Part model, mm, in its own coordinate system. Give positions to 0.01 mm unless a question says otherwise; leave off trailing zeros. Order: outer loops, then holes, each group sorted by start corner. A loop starts at its lowest first (then second) coordinate and runs counter-clockwise, first axis right, second up. Notation, with made-up numbers: M -30,51 L 19,51 A18 ccw 19,84 Z; hole C 50,51 d1. An arc over 180 degrees is marked long. Write each question's results on one line, items separated by ' | '. Start each with the question number.
from build123d import *

# Parameters (mm, degrees)
SKETCH1_R             = 41.5
MAIN_PLATE_DEPTH      = 5
SKETCH2_R             = 2.05
CUT_EXTRUDE_G27_DEPTH = 59.902461748
SKETCH3_R             = 2.5
MOMO_SPARKO_DEPTH     = 59.902461748
SKETCH4_R             = 17.5
CENTER_HOLE_DEPTH     = 59.902461748
FILLET1_R             = 2
FILLET2_R             = 2


with BuildPart() as part:
    # Sketch1 → Main Plate (new body)
    with BuildSketch(Plane(origin=(0, 0, 0), x_dir=(1, 0, 0), z_dir=(0, 1, 0))):
        with Locations(Location((0, 0, 0), (0, 0, 270))):
            Circle(SKETCH1_R)
    extrude(amount=MAIN_PLATE_DEPTH)

    # Sketch2 → Cut-Extrude G27 (cut, through all)
    with BuildSketch(Plane(origin=(0, 5, 0), x_dir=(1, 0, 0), z_dir=(0, 1, 0))):
        with Locations(Location((0, 27.5, 0), (0, 0, 270))):
            Circle(SKETCH2_R)
        with Locations(Location((23.815698604, 13.75, 0), (0, 0, 270))):
            Circle(SKETCH2_R)
        with Locations(Location((23.815698604, -13.75, 0), (0, 0, 270))):
            Circle(SKETCH2_R)
        with Locations(Location((0, -27.5, 0), (0, 0, 270))):
            Circle(SKETCH2_R)
        with Locations(Location((-23.815698604, -13.75, 0), (0, 0, 270))):
            Circle(SKETCH2_R)
        with Locations(Location((-23.815698604, 13.75, 0), (0, 0, 270))):
            Circle(SKETCH2_R)
    extrude(amount=-CUT_EXTRUDE_G27_DEPTH, mode=Mode.SUBTRACT)

    # Sketch3 → Momo - Sparko (cut, through all)
    with BuildSketch(Plane(origin=(0, 5, 0), x_dir=(1, 0, 0), z_dir=(0, 1, 0))):
        with Locations(Location((0, 35, 0), (0, 0, 270))):
            Circle(SKETCH3_R)
        with Locations(Location((30.310889132, 17.5, 0), (0, 0, 270))):
            Circle(SKETCH3_R)
        with Locations(Location((30.310889132, -17.5, 0), (0, 0, 270))):
            Circle(SKETCH3_R)
        with Locations(Location((0, -35, 0), (0, 0, 270))):
            Circle(SKETCH3_R)
        with Locations(Location((-30.310889132, -17.5, 0), (0, 0, 270))):
            Circle(SKETCH3_R)
        with Locations(Location((-30.310889132, 17.5, 0), (0, 0, 270))):
            Circle(SKETCH3_R)
    extrude(amount=-MOMO_SPARKO_DEPTH, mode=Mode.SUBTRACT)

    # Sketch4 → Center Hole (cut, through all)
    with BuildSketch(Plane(origin=(0, 5, 0), x_dir=(1, 0, 0), z_dir=(0, 1, 0))):
        with Locations(Location((0, 0, 0), (0, 0, 270))):
            Circle(SKETCH4_R)
    extrude(amount=-CENTER_HOLE_DEPTH, mode=Mode.SUBTRACT)

    # Fillet1
    fillet1_edges = [part.edges().sort_by_distance(p)[0] for p in [
        (0, 5, -41.5),
    ]]
    fillet(fillet1_edges, radius=FILLET1_R)

    # Fillet2
    fillet2_edges = [part.edges().sort_by_distance(p)[0] for p in [
        (0, 0, -41.5),
    ]]
    fillet(fillet2_edges, radius=FILLET2_R)


solid = part.part
(1) Drop flat-ended pins along their axis: P1, Ø1.5, axis at x = 29, y = 3.5, coming from the +Z side; P2, Ø8, axis at x = 0, z = -35, coming from the -Y side. Give the stop position or say it passes through.
(2) Probe L1, parallel to Z at x = -24.5, y = 4.3; L2, parallel to Z at x = -1.5, y = 1.9; L3, parallel to Z at x = -12, y = 4.75. List the from-to ranges inside material, lowest first.
(3) Saw through at B-B on x = 0. Give the cut face in (y, z).
(4) Saw through at A-A on z = 0. Give the cut face in (x, y), plus the area to 3 significant figures.
(5) Saw through at C-C on x = -31.5. Give the number of separate pieces and of enclosed holes in the cut face, plus the area to 3 significant figures.
(6) Pull direction Z, two halves, no side cores. Call faces 1 (the cylindrical face through (-32.75, 2.54, 16.96)), 2 (the cylindrical face through (12.465, 2.493, 39.584)), 3 (the flat face through (-8, 0, 17)): +Z half, -Z half, draft (parallel to the pull), parting line (faces both ways), or undercut.
Taken from the geometry:
1) P1: stops at z = 30.34 | P2: stops at y = 0
2) L1: z = -32.9 to -15.68, -11.82 to 11.82, 15.68 to 32.9 | L2: z = -41.47 to -37, -33 to -28.9, -26.1 to -17.44, 17.44 to 26.1, 28.9 to 33, 37 to 41.47 | L3: z = -38.65 to -12.74, 12.74 to 38.65
3) outline: M 0,-39.5 A2 ccw 2,-41.5 L 3,-41.5 A2 ccw 5,-39.5 L 5,-37.5 L 0,-37.5 Z; M 0,-32.5 L 5,-32.5 L 5,-29.55 L 0,-29.55 Z; M 0,-25.45 L 5,-25.45 L 5,-17.5 L 0,-17.5 Z; M 0,17.5 L 5,17.5 L 5,25.45 L 0,25.45 Z; M 0,29.55 L 5,29.55 L 5,32.5 L 0,32.5 Z; M 0,37.5 L 5,37.5 L 5,39.5 A2 ccw 3,41.5 L 2,41.5 A2 ccw 0,39.5 Z
4) outline: M -41.5,2 A2 ccw -39.5,0 L -17.5,0 L -17.5,5 L -39.5,5 A2 ccw -41.5,3 Z; M 17.5,0 L 39.5,0 A2 ccw 41.5,2 L 41.5,3 A2 ccw 39.5,5 L 17.5,5 Z | area: 237 mm²
5) separate pieces: 3 | enclosed holes: 0 | area: 221 mm²
6) face 1: undercut | face 2: parting line | face 3: draft
